The model under review builds one solid part; all positions refer to its coordinate system, in mm. A direction names the side the tool comes from. Coordinates: 2 decimals unless noted, no trailing zeros. Write each loop counter-clockwise with the first axis right and the second up, starting at its lowest first coordinate (ties: lowest second). Pieces come first, ordered by that corner, then holes. Notation, with made-up numbers: (85, 59.25) - (91, 59.25) arc R29 ccw to (91, 93.25) - close; hole circle Ø4 at (8.25, 77). An arc over 180 degrees is marked (long way). Return JSON: item names as keys, results as strings. Group by question number.
(1) We need section B-B on y = 74. State the section outline as (x, z) points, then the cut area to 3 significant figures.
(2) Tool access review of faces 1 (the face through (-0.91, 110.51, 0.7)), 2 (the face through (-1.08, 31.57, 4.88)): name each direction out of +Z, -Z, +X, -X, +Y, -Y from which nothing blocks a thin tool from reaching the whole face with its end or side.
(3) To check wall thickness, follow L1, parallel to X at y = -4.5, z = -0.5; L2, parallel to Z at x = 0.25, y = 73. State the ranges of each line that lie inside material, in increasing order. Write a range as from..to.
(4) We need section A-A on y = 12. State the section outline as (x, z) points.
(5) For pin 1 Ø1 at (x, y) = (1, 9) entering from +Z; pin 2 Ø6 at (x, y) = (2, 95.5) entering from +Z; pin 3 Ø3 at (y, z) = (44, 2) entering from -X, all flat-tipped, find the tip position at first contact; note any pin that passes through.
```python
from build123d import *

# Parameters (mm, degrees)
CHAMFER_1_SIZE = 0.5


# Read off the part's stored shape, not the designer's step: 旋转1
with BuildPart() as part:
    # 旋转1 outline → 旋转1 (revolve)
    with BuildSketch(Plane.XY):
        Polygon((1.15, 111.197298964), (0, 114.397298964), (0, -10.602701036), (5, -10.602701036), (5, 72.097298964), (4.6, 72.097298964), (4.6, 95.497298964), (3.6, 96.497298964), (3.6, 97.497298964), (1.55, 109.797298964), (1.15, 109.797298964), align=None)
    revolve(axis=Axis((0, 0, 0), (0, 1, 0)))

    # 倒角1
    chamfer_1_edges = [part.edges().sort_by_distance(p)[0] for p in [
        (-5, -10.602701036, 0),
    ]]
    chamfer(chamfer_1_edges, length=CHAMFER_1_SIZE)


solid = part.part
```
Ans:
{
 "1": {"outline": "circle Ø9.2 at (0, 0)", "area": "66.5 mm²"},
 "2": {"face 1": "+Y", "face 2": "+Y, -Y"},
 "3": {"L1": "-4.97..4.97", "L2": "-4.59..4.59"},
 "4": {"outline": "circle Ø10 at (0, 0)"},
 "5": {"pin 1": "z = 4.97", "pin 2": "z = 4.6", "pin 3": "x = -4.97"}
}
